Verification items for the finished model (mm, model axes). A direction names the side the tool comes from. Give positions to 0.01 mm unless a question says otherwise; leave off trailing zeros. Loops run counter-clockwise (first coordinate to the right, second up) from the corner with the lowest first, then second, coordinate; pieces in that order, holes last. Notation, with made-up numbers: (72, 2.5) - (124, 2.5) arc R18 ccw to (124, 34.5) - close; hole circle Ø8 at (46.5, -20.5). An arc over 180 degrees is marked (long way). Use one line per item in the form item = value.
```python
from build123d import *

# Parameters (mm, degrees)
F0_W          = 63.5
F0_H          = 95.25
F1_DEPTH      = 2.54
F2_R          = 5.08
F4_DEPTH      = 2.541
F6_DEPTH      = 2.54
F7_DEPTH      = 2.54
F7_DEPTH_BACK = 3.81


with BuildPart() as f1:
    # F0 (on Top) → F1 (new body)
    with BuildSketch(Plane.XY):
        with Locations((-31.75, 47.625)):
            Rectangle(F0_W, F0_H)
    extrude(amount=F1_DEPTH)

    # F2
    f2_edges = [f1.edges().sort_by_distance(p)[0] for p in [
        (-63.5, 0, 1.27),
        (0, 0, 1.27),
        (0, 95.25, 1.27),
        (-63.5, 95.25, 1.27),
    ]]
    fillet(f2_edges, radius=F2_R)

    # F3 (on face) → F4 (cut, through all)
    with BuildSketch(Plane.XY.offset(2.54)):
        with BuildLine():
            ThreePointArc((-28.7147323039, 56.4319934356), (-23.3894818135, 60.6365886522), (-18.0642313231, 56.4319934356))
            Line((-18.0642313231, 56.4319934356), (-16.1628100576, 56.4319934356))
            ThreePointArc((-16.1628100576, 56.4319934356), (-23.3894818135, 62.4994101926), (-30.6161535693, 56.4319934356))
            Line((-30.6161535693, 56.4319934356), (-28.7147323039, 56.4319934356))
        make_face()
        with BuildLine():
            Line((-16.1628100576, 53.8919934356), (-18.0642313231, 53.8919934356))
            ThreePointArc((-18.0642313231, 53.8919934356), (-23.3894818135, 49.687398219), (-28.7147323039, 53.8919934356))
            Line((-28.7147323039, 53.8919934356), (-30.6161535693, 53.8919934356))
            ThreePointArc((-30.6161535693, 53.8919934356), (-23.3894818135, 47.8245766785), (-16.1628100576, 53.8919934356))
        make_face()
        with BuildLine():
            ThreePointArc((-61.2091943622, 39.8156233132), (-3.7930509667, 50.3538420797), (-62.1665790677, 49.9079786241))
            Line((-62.1665790677, 49.9079786241), (-46.5377829969, 43.5084439814))
            ThreePointArc((-46.5377829969, 43.5084439814), (-44.1355102318, 44.6498304086), (-41.4878092706, 44.9015386403))
            Line((-41.4878092706, 44.9015386403), (-34.3481898308, 55.0450235605))
            ThreePointArc((-34.3481898308, 55.0450235605), (-15.6087357363, 62.8799564987), (-23.5952306539, 44.2045927048))
            Line((-23.5952306539, 44.2045927048), (-33.5741378367, 37.2411757708))
            ThreePointArc((-33.5741378367, 37.2411757708), (-40.8213137183, 28.6976707936), (-49.9820448458, 35.1470150054))
            Line((-49.9820448458, 35.1470150054), (-61.2091943622, 39.8156233132))
        make_face()
        with BuildLine():
            ThreePointArc((-47.366052866, 34.1452620924), (-36.0821241079, 34.4932892416), (-43.9929661581, 42.5472788847))
            Line((-43.9929661581, 42.5472788847), (-40.4547355891, 41.0624451561))
            ThreePointArc((-40.4547355891, 41.0624451561), (-37.8743531006, 35.1484300856), (-43.827822297, 32.6604283638))
            Line((-43.827822297, 32.6604283638), (-47.366052866, 34.1452620924))
        make_face()
    extrude(amount=-F4_DEPTH, mode=Mode.SUBTRACT)

    # F5 (on face) → F6 (join)
    with BuildSketch(Plane(origin=(0, 0, 0), x_dir=(1, 0, 0), z_dir=(0, 0, -1))):
        with BuildLine():
            Line((-63.5, -86.36), (-63.5, -83.82))
            Line((-63.5, -83.82), (-67.31, -83.82))
            ThreePointArc((-67.31, -83.82), (-66.4119743879, -84.1919743879), (-66.04, -85.09))
            ThreePointArc((-66.04, -85.09), (-66.4119743879, -85.9880256121), (-67.31, -86.36))
            Line((-67.31, -86.36), (-63.5, -86.36))
        make_face()
        with BuildLine():
            Line((-63.5, -63.5), (-63.5, -60.96))
            Line((-63.5, -60.96), (-67.31, -60.96))
            ThreePointArc((-67.31, -60.96), (-66.4119743879, -61.3319743879), (-66.04, -62.23))
            ThreePointArc((-66.04, -62.23), (-66.4119743879, -63.1280256121), (-67.31, -63.5))
            Line((-67.31, -63.5), (-63.5, -63.5))
        make_face()
        with BuildLine():
            Line((-63.5, -34.29), (-63.5, -31.75))
            Line((-63.5, -31.75), (-67.31, -31.75))
            ThreePointArc((-67.31, -31.75), (-66.4119743879, -32.1219743879), (-66.04, -33.02))
            ThreePointArc((-66.04, -33.02), (-66.4119743879, -33.9180256121), (-67.31, -34.29))
            Line((-67.31, -34.29), (-63.5, -34.29))
        make_face()
        with BuildLine():
            ThreePointArc((-67.31, -8.89), (-66.4119743879, -9.2619743879), (-66.04, -10.16))
            ThreePointArc((-66.04, -10.16), (-66.4119743879, -11.0580256121), (-67.31, -11.43))
            Line((-67.31, -11.43), (-63.5, -11.43))
            Line((-63.5, -11.43), (-63.5, -8.89))
            Line((-63.5, -8.89), (-67.31, -8.89))
        make_face()
        with BuildLine():
            Line((3.81, -8.89), (0, -8.89))
            Line((0, -8.89), (0, -11.43))
            Line((0, -11.43), (3.81, -11.43))
            ThreePointArc((3.81, -11.43), (2.54, -10.16), (3.81, -8.89))
        make_face()
        with BuildLine():
            Line((3.81, -31.75), (0, -31.75))
            Line((0, -31.75), (0, -34.29))
            Line((0, -34.29), (3.81, -34.29))
            ThreePointArc((3.81, -34.29), (2.54, -33.02), (3.81, -31.75))
        make_face()
        with BuildLine():
            Line((3.81, -60.96), (0, -60.96))
            Line((0, -60.96), (0, -63.5))
            Line((0, -63.5), (3.81, -63.5))
            ThreePointArc((3.81, -63.5), (2.54, -62.23), (3.81, -60.96))
        make_face()
        with BuildLine():
            Line((3.81, -83.82), (0, -83.82))
            Line((0, -83.82), (0, -86.36))
            Line((0, -86.36), (3.81, -86.36))
            ThreePointArc((3.81, -86.36), (2.54, -85.09), (3.81, -83.82))
        make_face()
    extrude(amount=-F6_DEPTH)

    # F5 (on face) → F7 (join, two sides)
    with BuildSketch(Plane(origin=(0, 0, 0), x_dir=(1, 0, 0), z_dir=(0, 0, -1))) as f7_sk:
        with BuildLine():
            ThreePointArc((-66.04, -85.09), (-66.4119743879, -84.1919743879), (-67.31, -83.82))
            ThreePointArc((-67.31, -83.82), (-68.58, -85.09), (-67.31, -86.36))
            ThreePointArc((-67.31, -86.36), (-66.4119743879, -85.9880256121), (-66.04, -85.09))
        make_face()
        with BuildLine():
            ThreePointArc((-66.04, -62.23), (-66.4119743879, -61.3319743879), (-67.31, -60.96))
            ThreePointArc((-67.31, -60.96), (-68.58, -62.23), (-67.31, -63.5))
            ThreePointArc((-67.31, -63.5), (-66.4119743879, -63.1280256121), (-66.04, -62.23))
        make_face()
        with BuildLine():
            ThreePointArc((-66.04, -33.02), (-66.4119743879, -32.1219743879), (-67.31, -31.75))
            ThreePointArc((-67.31, -31.75), (-68.58, -33.02), (-67.31, -34.29))
            ThreePointArc((-67.31, -34.29), (-66.4119743879, -33.9180256121), (-66.04, -33.02))
        make_face()
        with BuildLine():
            ThreePointArc((-67.31, -11.43), (-66.4119743879, -11.0580256121), (-66.04, -10.16))
            ThreePointArc((-66.04, -10.16), (-66.4119743879, -9.2619743879), (-67.31, -8.89))
            ThreePointArc((-67.31, -8.89), (-68.58, -10.16), (-67.31, -11.43))
        make_face()
        with BuildLine():
            ThreePointArc((5.08, -10.16), (4.7080256121, -9.2619743879), (3.81, -8.89))
            ThreePointArc((3.81, -8.89), (2.54, -10.16), (3.81, -11.43))
            ThreePointArc((3.81, -11.43), (4.7080256121, -11.0580256121), (5.08, -10.16))
        make_face()
        with BuildLine():
            ThreePointArc((5.08, -33.02), (4.7080256121, -32.1219743879), (3.81, -31.75))
            ThreePointArc((3.81, -31.75), (2.54, -33.02), (3.81, -34.29))
            ThreePointArc((3.81, -34.29), (4.7080256121, -33.9180256121), (5.08, -33.02))
        make_face()
        with BuildLine():
            ThreePointArc((5.08, -62.23), (4.7080256121, -61.3319743879), (3.81, -60.96))
            ThreePointArc((3.81, -60.96), (2.54, -62.23), (3.81, -63.5))
            ThreePointArc((3.81, -63.5), (4.7080256121, -63.1280256121), (5.08, -62.23))
        make_face()
        with BuildLine():
            ThreePointArc((5.08, -85.09), (4.7080256121, -84.1919743879), (3.81, -83.82))
            ThreePointArc((3.81, -83.82), (2.54, -85.09), (3.81, -86.36))
            ThreePointArc((3.81, -86.36), (4.7080256121, -85.9880256121), (5.08, -85.09))
        make_face()
    extrude(amount=-F7_DEPTH)
    extrude(f7_sk.sketch, amount=F7_DEPTH_BACK)


solid = f1.part
```
1. Draft check along X on faces 4 (the flat face through (0, 21, 1)), 5 (the cylindrical face through (-62.051, 93.722, 1.288)), 6 (the cylindrical face through (-36.16, 34.31, 1.29)), 7 (the flat face through (-65, 83.82, 1)). Enter one of: released by +X, released by -X, zero draft, split by the parting line, or undercut.
Result set:
face_4 = released by +X
face_5 = released by -X
face_6 = undercut
face_7 = zero draft
2. Tool access check on faces 1 (the cylindrical face through (-40.65, 28.72, 1.29)), 2 (the flat face through (2, 60.96, 1)), 3 (the flat face through (-63.5, 74, 1)). Record the directions out of +Z, -Z, +X, -X, +Y, -Y that give a thin tool (end or side, any length) a straight path to the whole face; none if there is none.
Result set:
face_1 = +Z, -Z
face_2 = +Z, -Z, +X
face_3 = +Z, -Z, -X
3. Depth check by flat-ended pin: pin 1 Ø2 at (y, z) = (68.5, 0) entering from +X; pin 2 Ø1.3 at (x, z) = (-65.5, 1.5) entering from -Y; pin 3 Ø0.8 at (x, z) = (-66, 1) entering from +Y. Enter the tip coordinate at first touch or a pass-through.
Result set:
pin_1 = 0
pin_2 = 8.89
pin_3 = 86.36
4. Section check D-D, the plane y = 51.5. Record the cut outline in (x, z), then the cut area to 3 significant figures.
Result set:
outline = (-63.5, 0) - (-62, 0) - (-62, 2.54) - (-63.5, 2.54) - close; (-36.84, 0) - (-29.75, 0) - (-29.75, 2.54) - (-36.84, 2.54) - close; (-27.46, 0) - (-19.32, 0) - (-19.32, 2.54) - (-27.46, 2.54) - close; (-17.03, 0) - (-13.06, 0) - (-13.06, 2.54) - (-17.03, 2.54) - close; (-3.92, 0) - (0, 0) - (0, 2.54) - (-3.92, 2.54) - close
area = 62.6 mm²
5. Section check A-A, the plane z = -1.25. Record the cut outline in (x, y), then the cut area to 3 significant figures.
Result set:
outline = circle Ø2.54 at (-67.31, 10.16); circle Ø2.54 at (-67.31, 33.02); circle Ø2.54 at (-67.31, 62.23); circle Ø2.54 at (-67.31, 85.09); circle Ø2.54 at (3.81, 10.16); circle Ø2.54 at (3.81, 33.02); circle Ø2.54 at (3.81, 62.23); circle Ø2.54 at (3.81, 85.09)
area = 40.5 mm²
6. Section check C-C, the plane y = 21. Record the cut outline in (x, z).
Result set:
outline = (-63.5, 0) - (-45.27, 0) - (-45.27, 2.54) - (-63.5, 2.54) - close; (-20.65, 0) - (0, 0) - (0, 2.54) - (-20.65, 2.54) - close
7. Section check B-B, the plane x = -56.5. Record the cut outline in (y, z), then the cut area to 3 significant figures.
Result set:
outline = (0, 0) - (30.14, 0) - (30.14, 2.54) - (0, 2.54) - close; (37.86, 0) - (47.59, 0) - (47.59, 2.54) - (37.86, 2.54) - close; (65.03, 0) - (95.25, 0) - (95.25, 2.54) - (65.03, 2.54) - close
area = 178 mm²
8. Scan lines: probe 1 along X at (y, z) = (38.5, 0.75); probe 2 along Y at (x, z) = (-43, 1.75); probe 3 along Y at (x, z) = (-32, 0.5). Record each from-to range of solid material in increasing order.
Result set:
probe_1 = -63.5 to -60.81, -58.05 to -37.87, -35.88 to -31.77, -5.11 to 0
probe_2 = 0 to 20.06, 28.71 to 30.75, 32.4 to 42.13, 42.83 to 44.87, 75.11 to 95.25
probe_3 = 0 to 18.3, 38.34 to 61.94, 76.87 to 95.25
